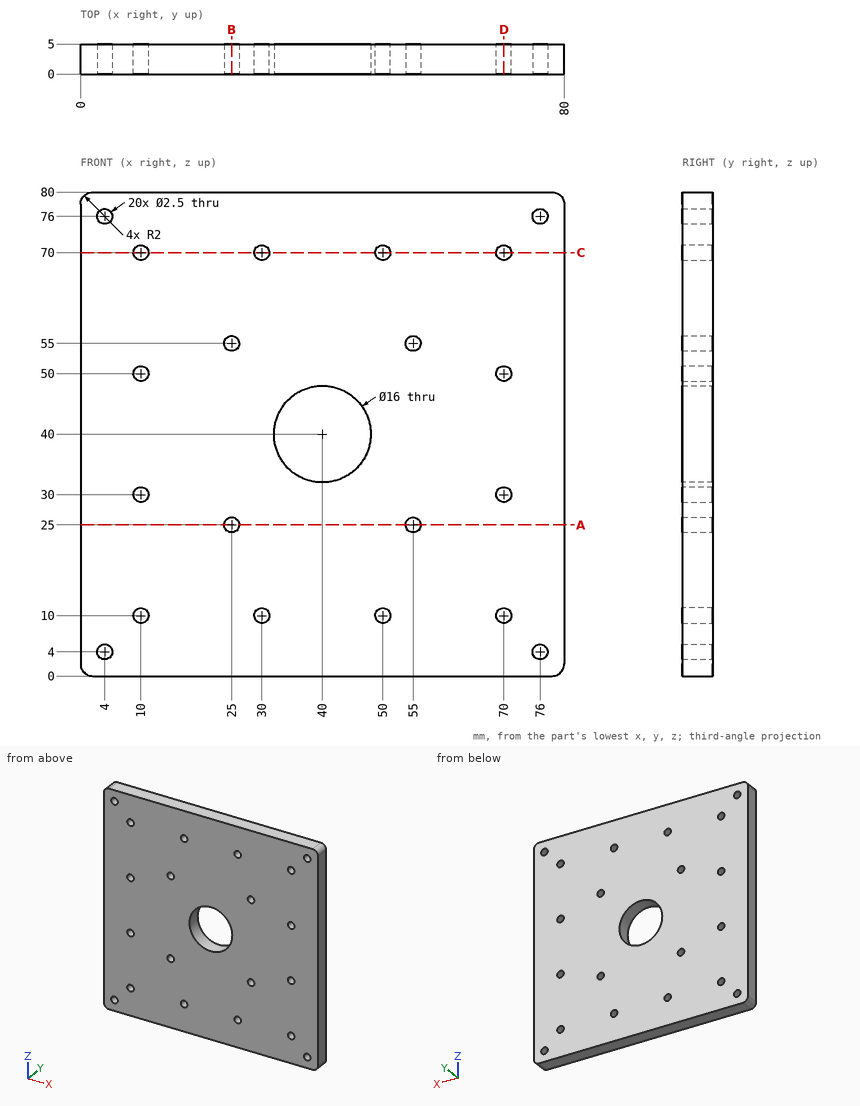
The drawing under review shows one solid part. Ordinate dimensions are in mm from its lowest x, y, z. Round coordinates to 2 decimals unless told otherwise and drop trailing zeros. Write each loop counter-clockwise with the first axis right and the second up, starting at its lowest first coordinate (ties: lowest second). Pieces come first, ordered by that corner, then holes. Notation, with made-up numbers: (83.5, 89) - (120.5, 89) arc R33 ccw to (120.5, 122) - close; hole circle Ø9 at (15, 47). An arc over 180 degrees is marked (long way). Write each question's results on one line, items separated by ' | '.
Item 1: Take a section at C-C on z = 70. State the section outline as (x, y) points, then the cut area to 3 significant figures.
Calculated:
outline: (0, 0) - (8.75, 0) - (8.75, 5) - (0, 5) - close; (11.25, 0) - (28.75, 0) - (28.75, 5) - (11.25, 5) - close; (31.25, 0) - (48.75, 0) - (48.75, 5) - (31.25, 5) - close; (51.25, 0) - (68.75, 0) - (68.75, 5) - (51.25, 5) - close; (71.25, 0) - (80, 0) - (80, 5) - (71.25, 5) - close | area: 350 mm^2
Item 2: Take a section at D-D on x = 70. State the section outline as (y, z) points, then the cut area to 3 significant figures.
Calculated:
outline: (0, 0) - (5, 0) - (5, 8.75) - (0, 8.75) - close; (0, 11.25) - (5, 11.25) - (5, 28.75) - (0, 28.75) - close; (0, 31.25) - (5, 31.25) - (5, 48.75) - (0, 48.75) - close; (0, 51.25) - (5, 51.25) - (5, 68.75) - (0, 68.75) - close; (0, 71.25) - (5, 71.25) - (5, 80) - (0, 80) - close | area: 350 mm^2
Item 3: To check wall thickness, follow line 1 along X through (y, z) = (2.75, 76); line 2 along X through (y, z) = (1.75, 70). State the ranges of each line that lie inside material, in increasing order. Write a range as from..to.
Calculated:
line 1: x = 0..2.75, 5.25..74.75, 77.25..80 | line 2: x = 0..8.75, 11.25..28.75, 31.25..48.75, 51.25..68.75, 71.25..80
Item 4: Take a section at B-B on x = 25. State the section outline as (y, z) points, then the cut area to 3 significant figures.
Calculated:
outline: (0, 0) - (5, 0) - (5, 23.75) - (0, 23.75) - close; (0, 26.25) - (5, 26.25) - (5, 53.75) - (0, 53.75) - close; (0, 56.25) - (5, 56.25) - (5, 80) - (0, 80) - close | area: 375 mm^2
Item 5: Take a section at A-A on z = 25. State the section outline as (x, y) points.
Calculated:
outline: (0, 0) - (23.75, 0) - (23.75, 5) - (0, 5) - close; (26.25, 0) - (53.75, 0) - (53.75, 5) - (26.25, 5) - close; (56.25, 0) - (80, 0) - (80, 5) - (56.25, 5) - close
